from build123d import *

# Parameters (mm, degrees)
SKETCH1_W           = 55
SKETCH1_H           = 95
BOSS_EXTRUDE1_DEPTH = 10
SKETCH3_W           = 52.6
SKETCH3_H           = 92.6
CUT_EXTRUDE1_DEPTH  = 8.8
FILLET1_R           = 2
CUT_EXTRUDE2_REACH  = 12
SKETCH4_R           = 5.5
CUT_EXTRUDE3_REACH  = 12
SKETCH5_R           = 5.5
SKETCH7_R           = 2.95
BOSS_EXTRUDE4_DEPTH = 20
CUT_EXTRUDE4_REACH  = 23.2
SKETCH8_R           = 1.75
BOSS_EXTRUDE5_DEPTH = 12
SKETCH11_R          = 2
BOSS_EXTRUDE6_DEPTH = 10
SKETCH12_R          = 0.75
CUT_EXTRUDE5_DEPTH  = 7


with BuildPart() as part:
    # Sketch1 → Boss-Extrude1 (new body)
    with BuildSketch(Plane(origin=(0, 0, 0), x_dir=(1, 0, 0), z_dir=(0, 1, 0))):
        with Locations((27.5, -47.5)):
            Rectangle(SKETCH1_W, SKETCH1_H)
    extrude(amount=-BOSS_EXTRUDE1_DEPTH)

    # Sketch3 → Cut-Extrude1 (cut)
    with BuildSketch(Plane.XZ.offset(10)):
        with Locations((27.5, 47.5)):
            Rectangle(SKETCH3_W, SKETCH3_H)
    extrude(amount=-CUT_EXTRUDE1_DEPTH, mode=Mode.SUBTRACT)

    # Fillet1
    fillet1_edges = [part.edges().sort_by_distance(p)[0] for p in [
        (0, -5, 0),
        (0, -5, 95),
        (55, -5, 95),
        (55, -5, 0),
    ]]
    fillet(fillet1_edges, radius=FILLET1_R)

    # Sketch4 → Cut-Extrude2 (cut, up to next)
    with BuildSketch(Plane(origin=(0, 0, 0), x_dir=(1, 0, 0), z_dir=(0, 1, 0)), mode=Mode.PRIVATE) as cut_extrude2_sk1:
        with Locations((42.8, -29.77)):
            Circle(SKETCH4_R)
    cut_extrude2_tool1 = extrude(cut_extrude2_sk1.sketch, amount=-CUT_EXTRUDE2_REACH, mode=Mode.PRIVATE) & part.part
    add(cut_extrude2_tool1.solids().sort_by_distance((42.8, 0, 29.77))[0], mode=Mode.SUBTRACT)
    # Sketch4 → Cut-Extrude2 (cut, up to next)
    with BuildSketch(Plane(origin=(0, 0, 0), x_dir=(1, 0, 0), z_dir=(0, 1, 0)), mode=Mode.PRIVATE) as cut_extrude2_sk2:
        with Locations((42.8, -19.28)):
            Circle(SKETCH4_R)
    cut_extrude2_tool2 = extrude(cut_extrude2_sk2.sketch, amount=-CUT_EXTRUDE2_REACH, mode=Mode.PRIVATE) & part.part
    add(cut_extrude2_tool2.solids().sort_by_distance((42.8, 0, 19.28))[0], mode=Mode.SUBTRACT)

    # Sketch5 → Cut-Extrude3 (cut, up to next)
    with BuildSketch(Plane(origin=(0, 0, 0), x_dir=(1, 0, 0), z_dir=(0, 1, 0)), mode=Mode.PRIVATE) as cut_extrude3_sk1:
        with Locations((12.2, -29.77)):
            Circle(SKETCH5_R)
    cut_extrude3_tool1 = extrude(cut_extrude3_sk1.sketch, amount=-CUT_EXTRUDE3_REACH, mode=Mode.PRIVATE) & part.part
    add(cut_extrude3_tool1.solids().sort_by_distance((12.2, 0, 29.77))[0], mode=Mode.SUBTRACT)
    # Sketch5 → Cut-Extrude3 (cut, up to next)
    with BuildSketch(Plane(origin=(0, 0, 0), x_dir=(1, 0, 0), z_dir=(0, 1, 0)), mode=Mode.PRIVATE) as cut_extrude3_sk2:
        with Locations((12.2, -19.28)):
            Circle(SKETCH5_R)
    cut_extrude3_tool2 = extrude(cut_extrude3_sk2.sketch, amount=-CUT_EXTRUDE3_REACH, mode=Mode.PRIVATE) & part.part
    add(cut_extrude3_tool2.solids().sort_by_distance((12.2, 0, 19.28))[0], mode=Mode.SUBTRACT)

    # Sketch7 → Boss-Extrude4 (add)
    with BuildSketch(Plane.XZ.offset(1.2)):
        with Locations((50.8, 88.2)):
            Circle(SKETCH7_R)
        with Locations((6.8, 88.2)):
            Circle(SKETCH7_R)
        with Locations((6.8, 4.2)):
            Circle(SKETCH7_R)
        with Locations((50.8, 4.2)):
            Circle(SKETCH7_R)
    extrude(amount=BOSS_EXTRUDE4_DEPTH)

    # Sketch8 → Cut-Extrude4 (cut, up to next)
    with BuildSketch(Plane(origin=(0, 0, 0), x_dir=(1, 0, 0), z_dir=(0, 1, 0)), mode=Mode.PRIVATE) as cut_extrude4_sk1:
        with Locations((6.8, -88.2)):
            Circle(SKETCH8_R)
    cut_extrude4_tool1 = extrude(cut_extrude4_sk1.sketch, amount=-CUT_EXTRUDE4_REACH, mode=Mode.PRIVATE) & part.part
    add(cut_extrude4_tool1.solids().sort_by_distance((6.8, 0, 88.2))[0], mode=Mode.SUBTRACT)
    # Sketch8 → Cut-Extrude4 (cut, up to next)
    with BuildSketch(Plane(origin=(0, 0, 0), x_dir=(1, 0, 0), z_dir=(0, 1, 0)), mode=Mode.PRIVATE) as cut_extrude4_sk2:
        with Locations((50.8, -88.2)):
            Circle(SKETCH8_R)
    cut_extrude4_tool2 = extrude(cut_extrude4_sk2.sketch, amount=-CUT_EXTRUDE4_REACH, mode=Mode.PRIVATE) & part.part
    add(cut_extrude4_tool2.solids().sort_by_distance((50.8, 0, 88.2))[0], mode=Mode.SUBTRACT)
    # Sketch8 → Cut-Extrude4 (cut, up to next)
    with BuildSketch(Plane(origin=(0, 0, 0), x_dir=(1, 0, 0), z_dir=(0, 1, 0)), mode=Mode.PRIVATE) as cut_extrude4_sk3:
        with Locations((50.8, -4.2)):
            Circle(SKETCH8_R)
    cut_extrude4_tool3 = extrude(cut_extrude4_sk3.sketch, amount=-CUT_EXTRUDE4_REACH, mode=Mode.PRIVATE) & part.part
    add(cut_extrude4_tool3.solids().sort_by_distance((50.8, 0, 4.2))[0], mode=Mode.SUBTRACT)
    # Sketch8 → Cut-Extrude4 (cut, up to next)
    with BuildSketch(Plane(origin=(0, 0, 0), x_dir=(1, 0, 0), z_dir=(0, 1, 0)), mode=Mode.PRIVATE) as cut_extrude4_sk4:
        with Locations((6.8, -4.2)):
            Circle(SKETCH8_R)
    cut_extrude4_tool4 = extrude(cut_extrude4_sk4.sketch, amount=-CUT_EXTRUDE4_REACH, mode=Mode.PRIVATE) & part.part
    add(cut_extrude4_tool4.solids().sort_by_distance((6.8, 0, 4.2))[0], mode=Mode.SUBTRACT)

    # Sketch10 → Boss-Extrude5 (add)
    with BuildSketch(Plane.XZ.offset(1.2)):
        Polygon((1.2, 93.8), (1.2, 1.2), (16.2, 1.2), (16.2, 2.4), (2.4, 2.4), (2.4, 92.6), (52.6, 92.6), (52.6, 2.4), (38.8, 2.4), (38.8, 1.2), (53.8, 1.2), (53.8, 93.8), align=None)
    extrude(amount=BOSS_EXTRUDE5_DEPTH)

    # Sketch11 → Boss-Extrude6 (add)
    with BuildSketch(Plane.XZ.offset(1.2)):
        with Locations((12.2, 9.275)):
            Circle(SKETCH11_R)
        with Locations((42.8, 9.275)):
            Circle(SKETCH11_R)
        with Locations((12.2, 39.775)):
            Circle(SKETCH11_R)
        with Locations((42.8, 39.775)):
            Circle(SKETCH11_R)
    extrude(amount=BOSS_EXTRUDE6_DEPTH)

    # Sketch12 → Cut-Extrude5 (cut)
    with BuildSketch(Plane(origin=(0, -11.2, 0), x_dir=(-1, 0, 0), z_dir=(0, -1, 0))):
        with Locations((-42.8, -39.775)):
            Circle(SKETCH12_R)
        with Locations((-12.2, -39.775)):
            Circle(SKETCH12_R)
        with Locations((-42.8, -9.275)):
            Circle(SKETCH12_R)
        with Locations((-12.2, -9.275)):
            Circle(SKETCH12_R)
    extrude(amount=-CUT_EXTRUDE5_DEPTH, mode=Mode.SUBTRACT)


solid = part.part
Model file for the job. Use its own axes, mm. A direction names the side the tool comes from. Give positions to 0.01 mm unless a question says otherwise; leave off trailing zeros. Order: outer loops, then holes, each group sorted by start corner. A loop starts at its lowest first (then second) coordinate and runs counter-clockwise, first axis right, second up. Notation, with made-up numbers: M 66.25,-4.5 L 109.25,-4.5 A32 cw 109.25,23.5 Z; hole C 80.25,25.25 d8. An arc over 180 degrees is marked long. Write item = value, one per line.
Q1. Drill centre lines: line 1 (Z direction, x = 42.8, y = -8.5) (3 decimals); line 2 (X direction, y = -0.45, z = 29.77); line 3 (Z direction, x = 50.8, y = -6). Where is each one in solid material? Low to high. Write a range as [from, to].
Derived:
line_1 = [0, 2.4], [7.275, 8.525], [10.025, 11.275], [37.775, 39.025], [40.525, 41.775], [92.6, 95]
line_2 = [0, 6.7], [17.7, 37.3], [48.3, 55]
line_3 = [0, 2.45], [5.95, 7.15], [85.25, 86.45], [89.95, 91.15], [92.6, 95]
Q2. Flat gauge pins, fed straight in: pin 1 (1 mm diameter, centred on x = 36, y = -12, fed in from +Z); pin 2 (5 mm diameter, centred on x = 31, z = 64.5, fed in from -Y); pin 3 (3 mm diameter, centred on x = 50.8, z = 4.2, fed in from -Y); pin 4 (1.6 mm diameter, centred on x = 42.5, y = -12, fed in from -Z). Where does each tip first touch, or does it go through?
Derived:
pin_1 = 93.8
pin_2 = -1.2
pin_3 = through
pin_4 = 1.2
Q3. Cut at A-A, the plane y = -16.5. List the corners of the cut face in (x, z).
Derived:
outline = C 6.8,4.2 d5.9; C 6.8,88.2 d5.9; C 50.8,4.2 d5.9; C 50.8,88.2 d5.9; hole C 6.8,4.2 d3.5; hole C 6.8,88.2 d3.5; hole C 50.8,4.2 d3.5; hole C 50.8,88.2 d3.5
Q4. Tool access for faces 4 (the cylindrical face through (6.42, -10.45, 89.91)), 5 (the flat face through (44, -7, 2.4)), 6 (the flat face through (9, -12, 1.2)), 7 (the flat face through (28, -12, 93.8)), 8 (the cylindrical face through (0.57, -5.07, 94.4)): list every direction of +Z, -Z, +X, -X, +Y, -Y with a clear straight run to the whole face (end or side of a thin tool).
Derived:
face_4 = +Y, -Y
face_5 = -Y
face_6 = -Z, +X, -X, -Y
face_7 = +Z, +X, -X, -Y
face_8 = +Z, -X, +Y, -Y
Q5. Cut at D-D, the plane y = -6.25. Count the separate pieces of the cut face and the enclosed holes in it, then the cut area to 3 significant figures.
Derived:
separate_pieces = 6
enclosed_holes = 9
area = 766 mm2
Q6. Cut at C-C, the plane x = 50.8. List the corners of the cut face in (y, z), then the cut area to 3 significant figures.
Derived:
outline = M -21.2,1.25 L -13.2,1.25 L -13.2,1.2 L -10,1.2 L -10,0 L 0,0 L 0,2.45 L -21.2,2.45 Z; M -21.2,5.95 L 0,5.95 L 0,86.45 L -21.2,86.45 L -21.2,85.25 L -1.2,85.25 L -1.2,7.15 L -21.2,7.15 Z; M -21.2,89.95 L 0,89.95 L 0,95 L -10,95 L -10,93.8 L -13.2,93.8 L -13.2,92.6 L -1.2,92.6 L -1.2,91.15 L -21.2,91.15 Z
area = 238 mm2
Q7. Cut at B-B, the plane z = 19.28. List the corners of the cut face in (x, y), then the cut area to 3 significant figures.
Derived:
outline = M 0,-10 L 1.2,-10 L 1.2,-13.2 L 2.4,-13.2 L 2.4,-1.2 L 6.7,-1.2 L 6.7,0 L 0,0 Z; M 17.7,-1.2 L 37.3,-1.2 L 37.3,0 L 17.7,0 Z; M 48.3,-1.2 L 52.6,-1.2 L 52.6,-13.2 L 53.8,-13.2 L 53.8,-10 L 55,-10 L 55,0 L 48.3,0 Z
area = 89.5 mm2
Q8. Two-plate mould, pull along Z, no slides. Class faces 1 (the cylindrical face through (44.65, -6.13, 39.01)), 2 (the flat face through (27, -5, 0)), 3 (the flat face through (54, -10, 47)): pulls with the +Z half, pulls with the -Z half, needs draft (parallel to the pull), parting line crosses it, or undercut.
Derived:
face_1 = undercut
face_2 = pulls with the -Z half
face_3 = needs draft
